```python
from build123d import *

# Parameters (mm, degrees)
F0_R     = 58.42
F3_DEPTH = 152.4
F4_DEPTH = 114.3
F1_R     = 53.34
F5_DEPTH = 114.3
F2_R     = 50.8
F6_DEPTH = 152.4


with BuildPart() as f3:
    # F0 (on Top) → F3 (new body, symmetric)
    with BuildSketch(Plane.XY):
        Circle(F0_R)
    extrude(amount=F3_DEPTH, both=True)

    # F0 (on Top) → F4 (cut, symmetric)
    with BuildSketch(Plane.XY):
        Circle(F0_R)
    extrude(amount=F4_DEPTH, both=True, mode=Mode.SUBTRACT)

    # F1 (on Top) → F5 (join, symmetric)
    with BuildSketch(Plane.XY):
        Circle(F1_R)
    extrude(amount=F5_DEPTH, both=True)

    # F2 (on Top) → F6 (cut, symmetric)
    with BuildSketch(Plane.XY):
        Circle(F2_R)
    extrude(amount=F6_DEPTH, both=True, mode=Mode.SUBTRACT)


solid = f3.part
```
Work out the finished part from the listing and answer in its coordinate system (mm). A direction names the side the tool comes from. Coordinates: 2 decimals unless noted, no trailing zeros. Order: outer loops, then holes, each group sorted by start corner. A loop starts at its lowest first (then second) coordinate and runs counter-clockwise, first axis right, second up. Notation, with made-up numbers: (79, -27) - (135, -27) arc R4 cw to (135, -20) - close; hole circle Ø10 at (-5.5, 14.25). An arc over 180 degrees is marked (long way). Answer as a JSON object with one key per item and string values.
1. Find section D-D on z = -127.5. Determine the outline of the cut face in (x, y).
Output values:
{"outline": "circle Ø116.84 at (0, 0); hole circle Ø101.6 at (0, 0)"}
2. A tool of negligible diameter and unlimited length cuts with its end or side. For faces 4 (the face through (-6.944, 52.886, 1.6)), 5 (the face through (-11.012, -49.592, 2.134)), from which of +Z, -Z, +X, -X, +Y, -Y can it reach the whole face along a straight path? Write none if from no direction.
Output values:
{"face 4": "none", "face 5": "+Z, -Z"}
3. Each of these flat-tipped pins is pushed along its axis until it touches: P1, Ø4, axis at y = -27.5, z = -100, coming from the -X side; P2, Ø12, axis at x = 12.5, z = 51, coming from the -Y side; P3, Ø8, axis at x = 39, y = 29.5, coming from the +Z side; P4, Ø10, axis at y = -10.5, z = -5.5, coming from the +X side. Where does it stop, or does it pass through?
Output values:
{"P1": "stops at x = -46.85", "P2": "stops at y = -52.94", "P3": "stops at z = 152.4", "P4": "stops at x = 53.06"}
4. Find section C-C on z = 46.5. Determine the outline of the cut face in (x, y), plus the area to 3 significant figures.
Output values:
{"outline": "circle Ø106.68 at (0, 0); hole circle Ø101.6 at (0, 0)", "area": "831 mm²"}
5. Consider line 1 (Y direction, x = 0, z = -82); line 2 (Y direction, x = 10.5, z = -27); line 3 (X direction, y = 41.5, z = -98.5). Determine where each line is inside the solid, lowest interval first.
Output values:
{"line 1": "y = -53.34 to -50.8, 50.8 to 53.34", "line 2": "y = -52.3 to -49.7, 49.7 to 52.3", "line 3": "x = -33.51 to -29.3, 29.3 to 33.51"}
6. Find section A-A on y = 0. Determine the outline of the cut face in (x, z).
Output values:
{"outline": "(-58.42, -152.4) - (-50.8, -152.4) - (-50.8, 152.4) - (-58.42, 152.4) - (-58.42, 114.3) - (-53.34, 114.3) - (-53.34, -114.3) - (-58.42, -114.3) - close; (50.8, -152.4) - (58.42, -152.4) - (58.42, -114.3) - (53.34, -114.3) - (53.34, 114.3) - (58.42, 114.3) - (58.42, 152.4) - (50.8, 152.4) - close"}
7. The mould has two halves that part along Z. Classify faces 1 (the face through (-43.06, 39.48, -133.08)), 2 (the face through (-18, 48, 152.4)), 3 (the face through (26, -47, -114.3)): +Z half, -Z half, draft (parallel to the pull), parting line (faces both ways), or undercut.
Output values:
{"face 1": "draft", "face 2": "+Z half", "face 3": "undercut"}
